Check sheet for the modelled part. Datum: model origin and axes. Units: mm. A direction names the side the tool comes from. Give positions to 0.01 mm unless a question says otherwise; leave off trailing zeros. Write each loop counter-clockwise with the first axis right and the second up, starting at its lowest first coordinate (ties: lowest second). Pieces come first, ordered by that corner, then holes. Notation, with made-up numbers: (87.25, -38.75) -> (132.25, -38.75) arc R19 cw to (132.25, -12.75) -> close; hole circle Ø6 at (-35.75, -9.75). An arc over 180 degrees is marked (long way). Return JSON: item names as keys, results as strings.
from build123d import *

# Parameters (mm, degrees)
BOSS_EXTRUDE2_DEPTH      = 12
BOSS_EXTRUDE2_DEPTH_BACK = 12
SKETCH1_4_W              = 13
SKETCH1_4_H              = 6
BOSS_EXTRUDE3_DEPTH      = 6
BOSS_EXTRUDE3_DEPTH_BACK = 6
FILLET1_R                = 2
SKETCH2_R                = 2.5
CUT_EXTRUDE1_DEPTH       = 18
SKETCH4_R                = 4
CUT_EXTRUDE2_DEPTH       = 7
CUT_EXTRUDE2_DEPTH_BACK  = 45
SKETCH5_R                = 5
CUT_EXTRUDE3_DEPTH       = 35


with BuildPart() as part:
    # Sketch1 → Boss-Extrude2 (new body, two sides)
    with BuildSketch(Plane(origin=(0, 0, 0), x_dir=(0, 0, -1), z_dir=(1, 0, 0))) as boss_extrude2_sk:
        Polygon((10.922768667, 10), (10.922768667, 22), (-40.111460143, 22), (-53.111460143, 22), (-53.111460143, -22), (10.922768667, -22), (10.922768667, -10), (-31.111460143, -10), (-31.111460143, 10), align=None)
    extrude(amount=BOSS_EXTRUDE2_DEPTH)
    extrude(boss_extrude2_sk.sketch, amount=-BOSS_EXTRUDE2_DEPTH_BACK)

    # Sketch1<4> → Boss-Extrude3 (add, two sides)
    with BuildSketch(Plane(origin=(0, 0, 0), x_dir=(0, 0, -1), z_dir=(1, 0, 0))) as boss_extrude3_sk:
        with Locations((-46.611460143, 25)):
            Rectangle(SKETCH1_4_W, SKETCH1_4_H)
    extrude(amount=BOSS_EXTRUDE3_DEPTH)
    extrude(boss_extrude3_sk.sketch, amount=-BOSS_EXTRUDE3_DEPTH_BACK)

    # Fillet1
    fillet1_edges = [part.edges().sort_by_distance(p)[0] for p in [
        (-12, -16, -10.922768667),
        (0, 22, -10.922768667),
        (0, 10, -10.922768667),
        (0, 10, 31.111460143),
        (0, -10, 31.111460143),
        (0, -10, -10.922768667),
        (0, -22, -10.922768667),
        (-12, -10, 10.094345738),
        (-12, 0, 31.111460143),
        (12, 0, 53.111460143),
        (12, -22, 21.094345738),
        (12, -16, -10.922768667),
        (12, -10, 10.094345738),
        (12, 0, 31.111460143),
        (12, 16, -10.922768667),
        (-12, 10, 10.094345738),
        (12, 10, 10.094345738),
        (12, 22, 21.094345738),
        (-12, 16, -10.922768667),
        (-12, 22, 21.094345738),
        (0, 22, 40.111460143),
        (6, 22, 46.611460143),
        (-6, 22, 46.611460143),
        (-12, 0, 53.111460143),
        (-12, -22, 21.094345738),
    ]]
    fillet(fillet1_edges, radius=FILLET1_R)

    # Sketch2 → Cut-Extrude1 (cut)
    with BuildSketch(Plane(origin=(0, 28, 0), x_dir=(1, 0, 0), z_dir=(0, 1, 0))):
        with Locations((0, -46.611460143)):
            Circle(SKETCH2_R)
    extrude(amount=-CUT_EXTRUDE1_DEPTH, mode=Mode.SUBTRACT)

    # Sketch4 → Cut-Extrude2 (cut, two sides)
    with BuildSketch(Plane(origin=(0, 22, 0), x_dir=(1, 0, 0), z_dir=(0, 1, 0))) as cut_extrude2_sk:
        with Locations((0, -0.077231333)):
            Circle(SKETCH4_R)
    extrude(amount=CUT_EXTRUDE2_DEPTH, mode=Mode.SUBTRACT)
    extrude(cut_extrude2_sk.sketch, amount=-CUT_EXTRUDE2_DEPTH_BACK, mode=Mode.SUBTRACT)

    # Sketch5 → Cut-Extrude3 (cut)
    with BuildSketch(Plane.XY.offset(53.111460143)):
        Circle(SKETCH5_R)
    extrude(amount=-CUT_EXTRUDE3_DEPTH, mode=Mode.SUBTRACT)


solid = part.part
(1) Cross-section at A-A on x = 0. State how many separate pieces and enclosed holes the cut face has, then the cut area to 3 significant figures.
Reply:
{"separate pieces": "4", "enclosed holes": "0", "area": "1,550 mm^2"}
(2) Cross-section at C-C on y = 4. Enter the section's corners in (x, z), then the cut area to 3 significant figures.
Reply:
{"outline": "(-12, 33.11) arc R2 ccw to (-10, 31.11) -> (-3, 31.11) -> (-3, 53.11) -> (-10, 53.11) arc R2 ccw to (-12, 51.11) -> close; (3, 31.11) -> (10, 31.11) arc R2 ccw to (12, 33.11) -> (12, 51.11) arc R2 ccw to (10, 53.11) -> (3, 53.11) -> close", "area": "393 mm^2"}
(3) Cross-section at D-D on z = 45.5. Enter the section's corners in (x, y), then the cut area to 3 significant figures.
Reply:
{"outline": "(-12, -20) arc R2 ccw to (-10, -22) -> (10, -22) arc R2 ccw to (12, -20) -> (12, 20) arc R2 ccw to (10, 22) -> (8, 22) arc R2 cw to (6, 24) -> (6, 28) -> (2.24, 28) -> (2.24, 10) -> (-2.24, 10) -> (-2.24, 28) -> (-6, 28) -> (-6, 24) arc R2 cw to (-8, 22) -> (-10, 22) arc R2 ccw to (-12, 20) -> close; hole circle Ø10 at (0, 0)", "area": "967 mm^2"}
(4) Thickness scan on L1, parallel to Z at x = 0, y = 14.5; L2, parallel to Y at x = -2.5, z = 15; L3, parallel to Y at x = 0, z = 48.5. Record the ranges inside material, lowest first.
Reply:
{"L1": "-10.92 to -3.92, 4.08 to 44.11, 49.11 to 53.11", "L2": "-22 to -10, 10 to 22", "L3": "-22 to -5, 5 to 10"}
(5) Set-up check for faces 1 (the cylindrical face through (-0.14, -9.4, 30.54)), 2 (the cylindrical face through (-11.43, -15.94, -10.32)), 3 (the cylindrical face through (11.399, 0.112, 31.682)), 4 (the flat face through (6, 26, 47)), 5 (the flat face through (0, 10, 47)): record each of +Z, -Z, +X, -X, +Y, -Y from which the full face is reachable in a straight line by a thin tool's end or side.
Reply:
{"face 1": "-Z, +X, -X", "face 2": "-Z, -X, +Y, -Y", "face 3": "-Z, +X", "face 4": "+Z, -Z, +X, +Y", "face 5": "+Y"}
(6) Depth check by flat-ended pin: pin 1 Ø7 at (x, z) = (0, 0.08) entering from -Y; pin 2 Ø1.2 at (y, z) = (25.5, 50) entering from +X; pin 3 Ø10 at (x, z) = (-1, 23.5) entering from +Y; pin 4 Ø5 at (x, y) = (4, 5.5) entering from -Z. Enter the tip coordinate at first touch or a pass-through.
Reply:
{"pin 1": "through", "pin 2": "x = 6", "pin 3": "y = 22", "pin 4": "z = 31.11"}
(7) Release check for a two-part mould opening along X. For faces 6 (the cylindrical face through (-11.43, 0.112, 31.713)), 7 (the cylindrical face through (-0.14, 10.57, -10.32)), 8 (the cylindrical face through (-1.08, -4.88, 42.27)) record: pulls with the +X half, pulls with the -X half, needs draft (parallel to the pull), parting line crosses it, or undercut.
Reply:
{"face 6": "pulls with the -X half", "face 7": "needs draft", "face 8": "undercut"}
(8) Cross-section at B-B on z = 14. Enter the section's corners in (x, y), then the cut area to 3 significant figures.
Reply:
{"outline": "(-12, -20) arc R2 ccw to (-10, -22) -> (10, -22) arc R2 ccw to (12, -20) -> (12, -12) arc R2 ccw to (10, -10) -> (-10, -10) arc R2 ccw to (-12, -12) -> close; (-12, 12) arc R2 ccw to (-10, 10) -> (10, 10) arc R2 ccw to (12, 12) -> (12, 20) arc R2 ccw to (10, 22) -> (-10, 22) arc R2 ccw to (-12, 20) -> close", "area": "569 mm^2"}
